Work out the finished part from the listing and answer in its coordinate system (mm). Face numbers are marked on the shaded views. Give positions to 0.01 mm unless a question says otherwise; leave off trailing zeros. Order: outer loops, then holes, each group sorted by start corner. A loop starts at its lowest first (then second) coordinate and runs counter-clockwise, first axis right, second up. Notation, with made-up numbers: (83, -4.75) - (101, -4.75) arc R28 cw to (101, 25.25) - close; hole circle Ø8 at (42, 29). An arc over 180 degrees is marked (long way). Write each question's results on one line, items separated by ' | '.
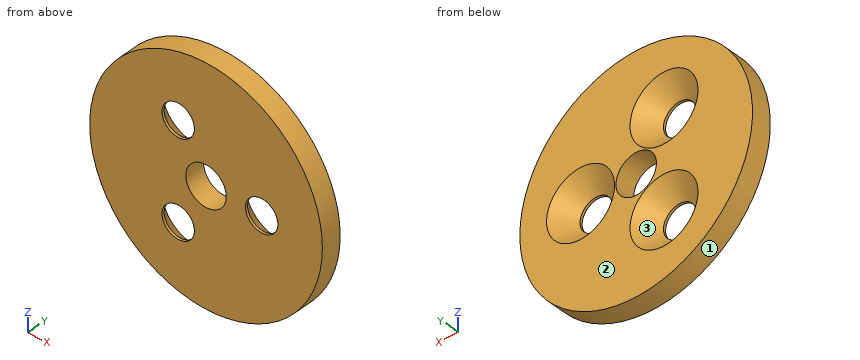
from build123d import *

# Parameters (mm, degrees)
SKIZZE1_R                          = 11.5
AUFSATZ_LINEAR_AUSTRAGEN1_DEPTH    = 2
KREISMUSTER1_COUNT                 = 3
F_4_0_4_DURCHMESSER_BOHRUNG1_D     = 4
F_4_0_4_DURCHMESSER_BOHRUNG1_DEPTH = 2


with BuildPart() as part:
    # Skizze1 → Aufsatz-Linear austragen1 (new body)
    with BuildSketch(Plane(origin=(0, 0, 0), x_dir=(1, 0, 0), z_dir=(0, 1, 0))):
        Circle(SKIZZE1_R)
    extrude(amount=AUFSATZ_LINEAR_AUSTRAGEN1_DEPTH)

    # Skizze2 → Formsenkung für M3 Senkschraube mit Innensechskant1 (revolve, cut)
    with BuildSketch(Plane(origin=(5.5, 2, 0), x_dir=(0, 0, 1), z_dir=(1, 0, 0))):
        Polygon((0, 0), (0, 2.001), (1.6, 2.001), (1.6, 1.76), (3.36, 0), align=None)
    formsenkung_f_r_m3_senkschraube_mit_inne = revolve(axis=Axis((5.5, 8.35, 0), (0, -1, 0)), mode=Mode.SUBTRACT)

    # Kreismuster1: Formsenkung für M3 Senkschraube mit Innensechskant1 ×3 about axis
    kreismuster1_axis = Axis((0, 0, 0), (0, 1, 0))
    for i in range(1, KREISMUSTER1_COUNT):
        add(formsenkung_f_r_m3_senkschraube_mit_inne.rotate(kreismuster1_axis, i * 360 / KREISMUSTER1_COUNT), mode=Mode.SUBTRACT)

    # Ø4.0 (4) Durchmesser Bohrung1
    with Locations(Plane(origin=(0, 2, 0), x_dir=(1, 0, 0), z_dir=(0, 1, 0))):
        with Locations((0, 0)):
            Hole(F_4_0_4_DURCHMESSER_BOHRUNG1_D / 2, depth=F_4_0_4_DURCHMESSER_BOHRUNG1_DEPTH)


solid = part.part
1. A cutting plane is placed at D-D, the plane y = 0.75. Write down the section's boundary in (x, z), then the cut area to 3 significant figures.
Answer list:
outline: circle Ø23 at (0, 0); hole circle Ø4.22 at (-2.75, -4.76); hole circle Ø4.22 at (-2.75, 4.76); hole circle Ø4 at (0, 0); hole circle Ø4.22 at (5.5, 0) | area: 361 mm^2
2. A cutting plane is placed at C-C, the plane x = -2.75. Write down the section's boundary in (y, z), then the cut area to 3 significant figures.
Answer list:
outline: (0, -11.17) - (2, -11.17) - (2, -8.12) - (0.24, -6.36) - (0, -6.36) - close; (0, -3.16) - (0.24, -3.16) - (2, -1.4) - (2, 1.4) - (0.24, 3.16) - (0, 3.16) - close; (0, 6.36) - (0.24, 6.36) - (2, 8.12) - (2, 11.17) - (0, 11.17) - close | area: 25.7 mm^2
3. A cutting plane is placed at B-B, the plane x = 5.5. Write down the section's boundary in (y, z).
Answer list:
outline: (0, -10.1) - (2, -10.1) - (2, -3.36) - (0.24, -1.6) - (0, -1.6) - close; (0, 1.6) - (0.24, 1.6) - (2, 3.36) - (2, 10.1) - (0, 10.1) - close
4. A cutting plane is placed at A-A, the plane z = 0. Write down the section's boundary in (x, y), then the cut area to 3 significant figures.
Answer list:
outline: (-11.5, 0) - (-2, 0) - (-2, 2) - (-11.5, 2) - close; (2, 0) - (3.9, 0) - (3.9, 0.24) - (2.14, 2) - (2, 2) - close; (7.1, 0) - (11.5, 0) - (11.5, 2) - (8.86, 2) - (7.1, 0.24) - close | area: 28.5 mm^2
5. Determine the mould class of the marked faces 1, 2 and 3 for opening direction Z: +Z half, -Z half, draft (parallel to the pull), parting line (faces both ways), or undercut.
Answer list:
face 1: parting line | face 2: draft | face 3: undercut
6. Given P1, Ø4, axis at x = 5.5, z = 0, coming from the +Y side; P2, Ø3.5, axis at x = -2.75, z = -4.76, coming from the +Y side; P3, Ø5, axis at x = -2.75, z = 4.76, coming from the +Y side, each flat-ended and moving along its own axis, determine where each tip first touches the part or whether it passes through.
Answer list:
P1: y = 0.64 | P2: y = 0.39 | P3: y = 1.14
7. Straight lines are drawn through the part: line 1 (Z direction, x = 0, y = 0.9); line 2 (Z direction, x = 5.5, y = 0.1); line 3 (X direction, y = 1.55, z = 2.25). For each, find the intervals that lie inside material, in ascending order. Write a range as [from, to].
Answer list:
line 1: [-11.5, -2], [2, 11.5] | line 2: [-10.1, -1.6], [1.6, 10.1] | line 3: [-11.28, -4.22], [-1.28, 3.65], [7.35, 11.28]
